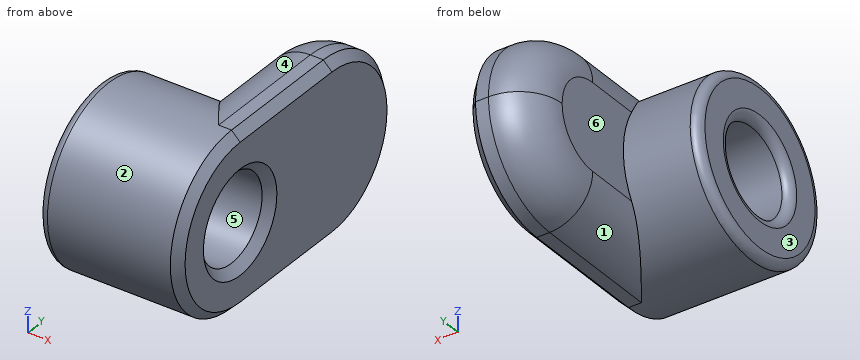
from build123d import *

# Parameters (mm, degrees)
SKETCH_1_R      = 4
SKETCH_1_R_2    = 2
EXTRUDE_1_DEPTH = 6.5
EXTRUDE_START   = -3
EXTRUDE_2_DEPTH = 3
FILLET_1_R      = 4
CHAMFER_1_SIZE  = 0.4
FILLET_2_R      = 2
FILLET_3_R      = 0.4


# Some blends are built 0.0001 mm under size
with BuildPart() as part:
    # 草图1 → 凸台-拉伸1 (new body)
    with BuildSketch(Plane(origin=(0, 0, 0), x_dir=(0, 0, -1), z_dir=(1, 0, 0))):
        with Locations(Location((0, 0, 0), (0, 0, 180))):
            Circle(SKETCH_1_R)
        with Locations(Location((0, 0, 0), (0, 0, 180))):
            Circle(SKETCH_1_R_2, mode=Mode.SUBTRACT)
    extrude(amount=EXTRUDE_1_DEPTH)

    # 草图2 → 凸台-拉伸2 (add)
    with BuildSketch(Plane(origin=(6.5, 0, 0), x_dir=(0, 0, -1), z_dir=(1, 0, 0)).offset(EXTRUDE_START)):
        with BuildLine():
            Line((2, 0), (4, 0))
            Line((4, 0), (4, 10))
            Line((4, 10), (-4, 10))
            Line((-4, 10), (-4, 0))
            Line((-4, 0), (-2, 0))
            ThreePointArc((-2, 0), (0, 2), (2, 0))
        make_face()
    extrude(amount=EXTRUDE_2_DEPTH)

    # 圆角1
    fillet_1_edges = [part.edges().sort_by_distance(p)[0] for p in [
        (5, 10, -4),
        (5, 10, 4),
    ]]
    fillet(fillet_1_edges, radius=FILLET_1_R - 0.0001)  # a hair under: the kernel refuses the full size

    # 倒角1
    chamfer_1_edges = [part.edges().sort_by_distance(p)[0] for p in [
        (6.5, -4, 0),
        (6.5, 3.00005, -4),
        (6.5, 3.00005, 4),
        (6.5, 8.828456414, 2.828456414),
        (6.5, 8.828456414, -2.828456414),
        (6.5, 0, -2),
    ]]
    chamfer(chamfer_1_edges, length=CHAMFER_1_SIZE)

    # 圆角2
    # the kernel refuses this fillet: 2 mm, written as the material it takes off along each edge
    with BuildSketch(Plane(origin=(3.5, -5, -4), x_dir=(0, 0, 1), z_dir=(0, 1, 0))) as fillet_2_piece_1_section:
        with BuildLine():
            CenterArc((FILLET_2_R, FILLET_2_R), FILLET_2_R, 180, 90)
            Line((0, FILLET_2_R), (0, 0))
            Line((0, 0), (FILLET_2_R, 0))
        make_face()
    fillet_2_piece_1 = extrude(amount=11.0001, mode=Mode.PRIVATE)
    fillet_2_piece_1 = fillet_2_piece_1 - Plane(origin=(4.073639318, 0, 0), x_dir=(0, 0, 1), z_dir=(-1, 0, 0)) * Cylinder(4, 31, mode=Mode.PRIVATE)
    add(fillet_2_piece_1, mode=Mode.SUBTRACT)
    with BuildSketch(Plane(origin=(3.5, 6.0001, 4), x_dir=(1, 0, 0), z_dir=(0, -1, 0))) as fillet_2_piece_2_section:
        with BuildLine():
            CenterArc((FILLET_2_R, -FILLET_2_R), FILLET_2_R, 90, 90)
            Line((0, -FILLET_2_R), (0, 0))
            Line((0, 0), (FILLET_2_R, 0))
        make_face()
    fillet_2_piece_2 = extrude(amount=11.0001, mode=Mode.PRIVATE)
    fillet_2_piece_2 = fillet_2_piece_2 - Plane(origin=(4.073638991, 0, 0), x_dir=(0, 0, 1), z_dir=(-1, 0, 0)) * Cylinder(4, 31, mode=Mode.PRIVATE)
    add(fillet_2_piece_2, mode=Mode.SUBTRACT)
    with BuildSketch(Plane(origin=(3.5, 6.0001, 0.0001), x_dir=(0, 0, 1), z_dir=(0, -1, 0))) as fillet_2_piece_3:
        with BuildLine():
            CenterArc((3.9999 - FILLET_2_R, -FILLET_2_R), FILLET_2_R, 0, 90)
            Line((3.9999 - FILLET_2_R, 0), (3.9999, 0))
            Line((3.9999, 0), (3.9999, -FILLET_2_R))
        make_face()
    revolve(axis=Axis((3.5, 6.0001, 0.0001), (-1, 0, 0)), revolution_arc=90, mode=Mode.SUBTRACT)
    with BuildSketch(Plane(origin=(3.5, 6.0001, -0.0001), x_dir=(0, 1, 0), z_dir=(0, 0, 1))) as fillet_2_piece_4:
        with BuildLine():
            CenterArc((3.9999 - FILLET_2_R, -FILLET_2_R), FILLET_2_R, 0, 90)
            Line((3.9999, -FILLET_2_R), (3.9999, 0))
            Line((3.9999, 0), (3.9999 - FILLET_2_R, 0))
        make_face()
    revolve(axis=Axis((3.5, 6.0001, -0.0001), (-1, 0, 0)), revolution_arc=90, mode=Mode.SUBTRACT)
    with BuildSketch(Plane(origin=(3.5, 10, -0.0001), x_dir=(0, -1, 0), z_dir=(0, 0, 1))) as fillet_2_piece_5:
        with BuildLine():
            CenterArc((FILLET_2_R, FILLET_2_R), FILLET_2_R, 180, 90)
            Line((0, FILLET_2_R), (0, 0))
            Line((0, 0), (FILLET_2_R, 0))
        make_face()
    extrude(amount=0.0002, mode=Mode.SUBTRACT)

    # 圆角3
    fillet_3_edges = [part.edges().sort_by_distance(p)[0] for p in [
        (0, 0, -4),
        (0, 0, -2),
    ]]
    fillet(fillet_3_edges, radius=FILLET_3_R)


solid = part.part
CAD build for the part. Positions are in the model's coordinates, mm. Face numbers are marked on the shaded views. A direction names the side the tool comes from. Give positions to 0.01 mm unless a question says otherwise; leave off trailing zeros. Write each loop counter-clockwise with the first axis right and the second up, starting at its lowest first coordinate (ties: lowest second). Pieces come first, ordered by that corner, then holes. Notation, with made-up numbers: (75, 39.25) -> (116, 39.25) arc R25 cw to (116, 73.25) -> close; hole circle Ø2 at (33, -31). An arc over 180 degrees is marked (long way). Return JSON: item names as keys, results as strings.
Item 1: Two-plate mould, pull along Z, no slides. Class the marked faces 4, 5 and 6: +Z half, -Z half, draft (parallel to the pull), parting line (faces both ways), or undercut.
Answer below:
{"face 4": "+Z half", "face 5": "undercut", "face 6": "draft"}
Item 2: Band-saw the part on A-A (x = 2.75). List the corners of the cut face in (y, z), then the cut area to 3 significant figures.
Answer below:
{"outline": "circle Ø8 at (0, 0); hole circle Ø4 at (0, 0)", "area": "37.7 mm2"}
Item 3: Drill centre lines: probe 1 along Y at (x, z) = (2.9, 0); probe 2 along Z at (x, y) = (0.5, -0.5); probe 3 along Z at (x, y) = (4.5, -1.25). Where is each one in solid material? Low to high.
Answer below:
{"probe 1": "y = -4 to -2, 2 to 4", "probe 2": "z = -3.97 to -1.94, 1.94 to 3.97", "probe 3": "z = -3.8 to -1.56, 1.56 to 3.8"}
Item 4: Drop flat-ended pins along their axis: pin 1 (1 mm diameter, centred on x = 4.5, y = 6, fed in from -Z); pin 2 (2 mm diameter, centred on y = 8.5, z = -3, fed in from -X); pin 3 (3 mm diameter, centred on y = 7, z = 0, fed in from -X). Give the stop position or say it passes through.
Answer below:
{"pin 1": "stops at z = -3.94", "pin 2": "stops at x = 3.72", "pin 3": "stops at x = 3.5"}
Item 5: Tool access for the marked faces 1, 2 and 3: list every direction of +Z, -Z, +X, -X, +Y, -Y with a clear straight run to the whole face (end or side of a thin tool).
Answer below:
{"face 1": "-Z, -X, +Y", "face 2": "-X", "face 3": "+Z, -Z, -X, +Y, -Y"}
